```python
from build123d import *

# Parameters (mm, degrees)
F1_DEPTH = 14
F3_DEPTH = 64
F4_R     = 12
F5_R     = 6
F6_DEPTH = 14


with BuildPart() as f1:
    # F0 (on Front) → F1 (new body)
    with BuildSketch(Plane.XZ):
        Polygon((0, 86.9015205713), (0, 0), (72, 0), (72, 45), (50.1107108272, 105.1403277303), align=None)
    extrude(amount=F1_DEPTH)

    # F2 (on face) → F3 (join, through all)
    with BuildSketch(Plane(origin=(-27.9296103431, 0, 76.7359737518), x_dir=(0.9396926208, 0, 0.3420201433), z_dir=(-0.3420201433, 0, 0.9396926208))):
        Polygon((83.0487751462, -14), (29.722070521, -14), (29.722070521, -82), (49.722070521, -82), (58.5238033349, -64.0408936895), (47.0034087749, -64.8243747139), (62.647170961, -32.9047522785), (69.0858827116, -42.4899661168), align=None)
    extrude(amount=-F3_DEPTH)

    # F4
    f4_edges = [f1.edges().sort_by_distance(p)[0] for p in [
        (0, -7, 0),
        (72, -7, 0),
    ]]
    fillet(f4_edges, radius=F4_R)

    # F5 (on face) → F6 (cut, through all)
    with BuildSketch(Plane.XZ.offset(14)):
        with Locations((12, 12)):
            Circle(F5_R)
        with Locations((60, 12)):
            Circle(F5_R)
    extrude(amount=-F6_DEPTH, mode=Mode.SUBTRACT)


solid = f1.part
```
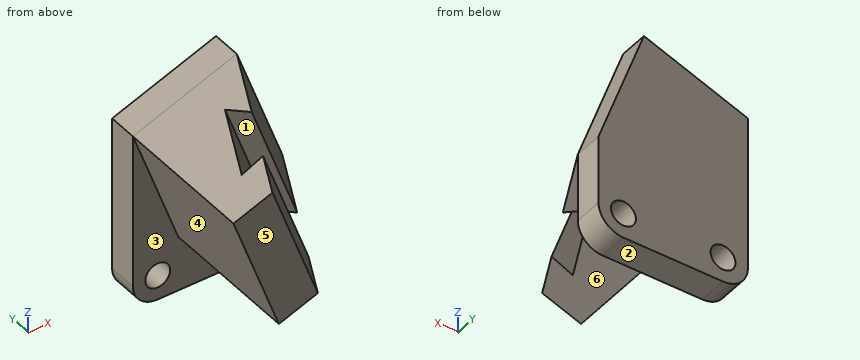
Geometry check sheet. Reference: the model listing, model coordinates, mm. Face numbers are marked on the shaded views. A direction names the side the tool comes from. Give positions to 0.01 mm unless a question says otherwise; leave off trailing zeros. Order: outer loops, then holes, each group sorted by start corner. A loop starts at its lowest first (then second) coordinate and runs counter-clockwise, first axis right, second up. Notation, with made-up numbers: (41, 49) - (63, 49) arc R16 cw to (63, 80) - close; hole circle Ø9 at (21.5, -7). An arc over 180 degrees is marked (long way). Write item = value, one per line. Start each with the question number.
1) Scan lines: L1, parallel to Y at x = 5, z = 16; L2, parallel to Z at x = 12, y = -6; L3, parallel to Y at x = 29.5, z = 81.5. Record each from-to range of solid material in increasing order.
2) Section check C-C (y = -70.5). Enter the section's corners in (x, z), then the cut area to 3 significant figures.
3) Section check A-A (z = 8.5). Enter the section's corners in (x, y), then the cut area to 3 significant figures.
4) Gauge pin test, flat ends, axial feed: pin 1 Ø1 at (y, z) = (-31.5, 27.5) entering from -X; pin 2 Ø11 at (x, z) = (60, 12) entering from -Y; pin 3 Ø2 at (y, z) = (-72, 56.5) entering from -X; pin 4 Ø4 at (x, y) = (11.5, -41.5) entering from +Z. Record the tip position at first contact, or that the pin passes through.
5) Section check D-D (z = 84.5). Enter the section's corners in (x, y).
6) Access from +Z, -Z, +X, -X, +Y, -Y to the whole of each face (thin tool, end or side, straight path). Record for the marked faces 4, 5 and 6.
7) Draft check along Z on the marked faces 1, 2 and 3. Enter one of: released by +Z, released by -Z, zero draft, split by the parting line, or undercut.
8) Section check B-B (z = 66). Enter the section's corners in (x, y).
Geometry check:
q1.L1 = -14 to 0
q1.L2 = 0 to 6, 18 to 91.27
q1.L3 = -70.02 to -64.24, -47.29 to 0
q2.outline = (0, 86.9) - (21.89, 26.76) - (45.98, 35.53) - (24.09, 95.67) - close
q2.area = 1,640 mm2
q3.outline = (0.52, -14) - (7.13, -14) - (7.13, 0) - (0.52, 0) - close; (16.87, -14) - (55.13, -14) - (55.13, 0) - (16.87, 0) - close; (64.87, -14) - (71.48, -14) - (71.48, 0) - (64.87, 0) - close
q3.area = 720 mm2
q4.pin_1 = 21.44
q4.pin_2 = through
q4.pin_3 = 10.7
q4.pin_4 = 91.82
q5.outline = (0, -14) - (0.87, -14) - (0.87, -82) - (22.16, -82) - (31.52, -64.04) - (19.26, -64.82) - (35.91, -32.9) - (42.76, -42.49) - (57.62, -14) - (57.62, 0) - (0, 0) - close
q6.face_4 = -Z, -X, -Y
q6.face_5 = +Z, -Z, +X, -X, -Y
q6.face_6 = -Z, +X, -Y
q7.face_1 = undercut
q7.face_2 = released by -Z
q7.face_3 = zero draft
q8.outline = (0, -14) - (7.61, -14) - (7.61, -82) - (28.89, -82) - (38.26, -64.04) - (26, -64.82) - (42.65, -32.9) - (49.5, -42.49) - (64.36, -14) - (64.36, 0) - (0, 0) - close
